The model under review builds one solid part; all positions refer to its coordinate system, in mm. A direction names the side the tool comes from. Round coordinates to 2 decimals unless told otherwise and drop trailing zeros.
1) Machinability: for faces 1 (the face through (-46.48, -0.78, 9.36)), 2 (the face through (-1, 0, -1)), which of the approach directions +Z, -Z, +X, -X, +Y, -Y give a long, thin tool a straight path to every point of the face, cutting with its end or side? Answer none if there is none.
2) To check wall thickness, follow L1, parallel to X at y = -1.05, z = 2.5; L2, parallel to X at y = -0.3, z = -3.5; L3, parallel to X at y = -1.45, z = -29. State the ranges of each line that lie inside material, in increasing order.
3) Mouldability with a two-part tool opening along X and no side actions: class faces 3 (the face through (-46.69, -0.78, -9.36)), 4 (the face through (69.329, -0.805, -49.895)), 5 (the face through (-68.511, -0.805, 49.845)), 6 (the face through (-42.34, -0.78, 30.01)) as pulls with the +X half, pulls with the -X half, needs draft (parallel to the pull), parting line crosses it, or undercut.
4) Clearance check with a flat-ended pin moving along its axis: P1, Ø2.5, axis at x = 43.71, z = -30.35, coming from the +Y side. State where the tip first meets the part, or that it passes through.
from build123d import *

# Parameters (mm, degrees)
SKETCH1_W           = 139.7
SKETCH1_H           = 101.6
BOSS_EXTRUDE1_DEPTH = 1.5875
SKETCH2_R           = 0.5
SKETCH2_R_2         = 1.5875
CUT_EXTRUDE1_DEPTH  = 87.735242522
CUT_EXTRUDE2_DEPTH  = 87.735242522
FILLET1_R           = 3.175


with BuildPart() as part:
    # Sketch1 → Boss-Extrude1 (new body)
    with BuildSketch(Plane(origin=(0, 0, 0), x_dir=(1, 0, 0), z_dir=(0, 1, 0))):
        with Locations((0.434010551, 0)):
            Rectangle(SKETCH1_W, SKETCH1_H)
    extrude(amount=-BOSS_EXTRUDE1_DEPTH)

    # Sketch2 → Cut-Extrude1 (cut, through all)
    with BuildSketch(Plane(origin=(0, 0, 0), x_dir=(1, 0, 0), z_dir=(0, 1, 0))):
        with Locations(Location((-51.22545, 24.505, 0), (0, 0, 270))):
            Circle(SKETCH2_R)
        with Locations(Location((-30.27045, 28.315, 0), (0, 0, 270))):
            Circle(SKETCH2_R)
        with Locations(Location((-30.27045, 32.125, 0), (0, 0, 270))):
            Circle(SKETCH2_R)
        with Locations(Location((-30.27045, -32.135, 0), (0, 0, 270))):
            Circle(SKETCH2_R)
        with Locations(Location((-30.27045, -28.325, 0), (0, 0, 270))):
            Circle(SKETCH2_R)
        with Locations(Location((-30.27045, -24.515, 0), (0, 0, 270))):
            Circle(SKETCH2_R)
        with Locations(Location((-30.27045, -20.705, 0), (0, 0, 270))):
            Circle(SKETCH2_R)
        with Locations(Location((51.47945, -6.483, 0), (0, 0, 270))):
            Circle(SKETCH2_R)
        with Locations(Location((51.47945, -2.673, 0), (0, 0, 270))):
            Circle(SKETCH2_R)
        with Locations(Location((-51.22545, 28.315, 0), (0, 0, 270))):
            Circle(SKETCH2_R)
        with Locations(Location((-51.22545, 32.125, 0), (0, 0, 270))):
            Circle(SKETCH2_R)
        with Locations(Location((-51.35245, -32.135, 0), (0, 0, 270))):
            Circle(SKETCH2_R)
        with Locations(Location((-51.35245, -28.325, 0), (0, 0, 270))):
            Circle(SKETCH2_R)
        with Locations(Location((-51.35245, -24.515, 0), (0, 0, 270))):
            Circle(SKETCH2_R)
        with Locations(Location((-51.35245, -20.705, 0), (0, 0, 270))):
            Circle(SKETCH2_R)
        with Locations(Location((-30.27045, 20.695, 0), (0, 0, 270))):
            Circle(SKETCH2_R)
        with Locations(Location((-30.27045, 24.505, 0), (0, 0, 270))):
            Circle(SKETCH2_R)
        with Locations(Location((-40.78945, -30.35, 0), (0, 0, 270))):
            Circle(SKETCH2_R_2)
        with Locations(Location((-40.78945, 30.35, 0), (0, 0, 270))):
            Circle(SKETCH2_R_2)
        with Locations(Location((43.71055, 30.35, 0), (0, 0, 270))):
            Circle(SKETCH2_R_2)
        with Locations(Location((43.71055, -30.35, 0), (0, 0, 270))):
            Circle(SKETCH2_R_2)
        with Locations(Location((51.47945, 1.137, 0), (0, 0, 270))):
            Circle(SKETCH2_R)
        with Locations(Location((-51.22545, 20.695, 0), (0, 0, 270))):
            Circle(SKETCH2_R)
    extrude(amount=-CUT_EXTRUDE1_DEPTH, mode=Mode.SUBTRACT)

    # Sketch3 → Cut-Extrude2 (cut, through all)
    with BuildSketch(Plane(origin=(0, 0, 0), x_dir=(1, 0, 0), z_dir=(0, 1, 0))):
        with BuildLine():
            Line((-41.912921413, 4.689952831), (-41.912921413, -4.689952831))
            ThreePointArc((-41.912921413, -4.689952831), (-46.582921413, -9.359952831), (-51.252921413, -4.689952831))
            Line((-51.252921413, -4.689952831), (-51.252921413, 4.689952831))
            ThreePointArc((-51.252921413, 4.689952831), (-46.582921413, 9.359952831), (-41.912921413, 4.689952831))
        make_face()
    extrude(amount=-CUT_EXTRUDE2_DEPTH, mode=Mode.SUBTRACT)

    # Fillet1
    fillet1_edges = [part.edges().sort_by_distance(p)[0] for p in [
        (70.284010551, -0.79375, 50.8),
        (-69.415989449, -0.79375, 50.8),
        (-69.415989449, -0.79375, -50.8),
        (70.284010551, -0.79375, -50.8),
    ]]
    fillet(fillet1_edges, radius=FILLET1_R)


solid = part.part
Answer below:
1. face 1: +Y, -Y
1. face 2: +Z, -Z, +X, -X, +Y
2. L1: x = -69.42 to -51.25, -41.91 to 51.01, 51.95 to 70.28
2. L2: x = -69.42 to -51.25, -41.91 to 70.28
2. L3: x = -69.42 to -41.62, -39.95 to 42.88, 44.55 to 70.28
3. face 3: undercut
3. face 4: pulls with the +X half
3. face 5: pulls with the -X half
3. face 6: undercut
4. P1: passes through
